Part model, mm, in its own coordinate system. A direction names the side the tool comes from. Round coordinates to 2 decimals unless told otherwise and drop trailing zeros. Order: outer loops, then holes, each group sorted by start corner. A loop starts at its lowest first (then second) coordinate and runs counter-clockwise, first axis right, second up. Notation, with made-up numbers: (59, 8.25) -> (86, 8.25) arc R15 cw to (86, 24.25) -> close; hole circle Ø3 at (-25.5, -29.5). An arc over 180 degrees is marked (long way). Answer as a JSON object with one key per item and string values. Group by question number.
```python
from build123d import *

# Parameters (mm, degrees)
F0_W     = 127
F0_H     = 72.898
F0_R     = 9.525
F0_H_2   = 168.402
F1_DEPTH = 79.502
F2_W     = 127
F2_H     = 72.898
F3_DEPTH = 57.15


with BuildPart() as f1:
    # F0 (on Top) → F1 (new body)
    with BuildSketch(Plane.XY):
        with Locations((63.5, 36.449)):
            Rectangle(F0_W, F0_H)
        with Locations((31.75, 35.052)):
            Circle(F0_R, mode=Mode.SUBTRACT)
        with Locations((63.5, 157.099)):
            Rectangle(F0_W, F0_H_2)
        with Locations((91.948, 114.3)):
            Circle(F0_R, mode=Mode.SUBTRACT)
        with Locations((31.75, 157.099)):
            Circle(F0_R, mode=Mode.SUBTRACT)
        with Locations((91.948, 199.898)):
            Circle(F0_R, mode=Mode.SUBTRACT)
    extrude(amount=F1_DEPTH)

    # F2 (on face) → F3 (cut)
    with BuildSketch(Plane.XY.offset(79.502)):
        with Locations((63.5, 36.449)):
            Rectangle(F2_W, F2_H)
    extrude(amount=-F3_DEPTH, mode=Mode.SUBTRACT)


solid = f1.part
```
Q1. Band-saw the part on B-B (y = 114.3). List the corners of the cut face in (x, z).
Q2. Band-saw the part on D-D (x = 117.5). List the corners of the cut face in (y, z).
Q3. Two-plate mould, pull along Y, no slides. Class faces 1 (the cylindrical face through (84.93, 120.74, 39.19)), 2 (the flat face through (63, 37, 22.352)), 3 (the flat face through (63, 0, 11)): +Y half, -Y half, draft (parallel to the pull), parting line (faces both ways), or undercut.
Q4. Band-saw the part on C-C (z = 15.5). List the corners of the cut face in (x, y) (3 decimals).
Q5. Which spindle directions (+Z, -Z, +X, -X, +Y, -Y) get a long thin tool onto all of the face, cutting with end or side? Do faces 4 (the flat face through (63, 122, 0)), 5 (the flat face through (63, 72.898, 51)). Say none if no direction does.
Q6. Band-saw the part on A-A (x = 31.75). List the corners of the cut face in (y, z), plus the area to 3 significant figures.
Q7. Wall check: line 1 (X direction, y = 114.5, z = 28); line 2 (Y direction, x = 58, z = 66.5); line 3 (Y direction, x = 26.5, z = 72). Give the ranges that are in metal, low to high. Write a range as [from, to].
Q8. Drop flat-ended pins along their axis: pin 1 Ø11.5 at (x, y) = (31.75, 157.099) entering from +Z; pin 2 Ø2 at (x, z) = (26, 27.5) entering from -Y. Give the stop position or say it passes through.
Completed:
{
 "1": {"outline": "(0, 0) -> (82.42, 0) -> (82.42, 79.5) -> (0, 79.5) -> close; (101.47, 0) -> (127, 0) -> (127, 79.5) -> (101.47, 79.5) -> close"},
 "2": {"outline": "(0, 0) -> (241.3, 0) -> (241.3, 79.5) -> (72.9, 79.5) -> (72.9, 22.35) -> (0, 22.35) -> close"},
 "3": {"face 1": "undercut", "face 2": "draft", "face 3": "-Y half"},
 "4": {"outline": "(0, 0) -> (127, 0) -> (127, 241.3) -> (0, 241.3) -> close; hole circle Ø19.05 at (31.75, 35.052); hole circle Ø19.05 at (31.75, 157.099); hole circle Ø19.05 at (91.948, 114.3); hole circle Ø19.05 at (91.948, 199.898)"},
 "5": {"face 4": "-Z, +X, -X, +Y, -Y", "face 5": "+Z, +X, -X, -Y"},
 "6": {"outline": "(0, 0) -> (25.53, 0) -> (25.53, 22.35) -> (0, 22.35) -> close; (44.58, 0) -> (147.57, 0) -> (147.57, 79.5) -> (72.9, 79.5) -> (72.9, 22.35) -> (44.58, 22.35) -> close; (166.62, 0) -> (241.3, 0) -> (241.3, 79.5) -> (166.62, 79.5) -> close", "area": "13,100 mm2"},
 "7": {"line 1": "[0, 82.43], [101.47, 127]", "line 2": "[72.9, 241.3]", "line 3": "[72.9, 149.15], [165.05, 241.3]"},
 "8": {"pin 1": "through", "pin 2": "y = 72.9"}
}
